```python
from build123d import *

# Parameters (mm, degrees)
SKETCH2_W           = 124.173
SKETCH2_H           = 119.38
BOSS_EXTRUDE1_DEPTH = 3.175
SKETCH4_R           = 1.905
CUT_EXTRUDE1_DEPTH  = 14.175
SKETCH10_W          = 1.59
SKETCH10_H          = 120
CUT_EXTRUDE3_DEPTH  = 10
SKETCH11_R          = 1.905
CUT_EXTRUDE4_DEPTH  = 10


with BuildPart() as part:
    # Sketch2 → Boss-Extrude1 (new body)
    with BuildSketch(Plane.XY):
        with Locations((40.767155738, -50.87039032)):
            Rectangle(SKETCH2_W, SKETCH2_H)
    extrude(amount=BOSS_EXTRUDE1_DEPTH)

    # Sketch4 → Cut-Extrude1 (cut)
    with BuildSketch(Plane.XY):
        with Locations((-15.867344262, -37.32039032)):
            Circle(SKETCH4_R)
        with Locations((-15.867344262, -64.42239032)):
            Circle(SKETCH4_R)
        with Locations((84.503655738, 3.36760968)):
            Circle(SKETCH4_R)
        with Locations((84.503655738, -105.10839032)):
            Circle(SKETCH4_R)
    extrude(amount=CUT_EXTRUDE1_DEPTH, mode=Mode.SUBTRACT)

    # Sketch10 → Cut-Extrude3 (cut)
    with BuildSketch(Plane(origin=(102.853655738, 0, 0), x_dir=(0, 0, -1), z_dir=(1, 0, 0))):
        with Locations((-2.380000064, -51.180389625)):
            Rectangle(SKETCH10_W, SKETCH10_H)
    extrude(amount=-CUT_EXTRUDE3_DEPTH, mode=Mode.SUBTRACT)

    # Sketch11 → Cut-Extrude4 (cut)
    with BuildSketch(Plane.XY.offset(1.585000064)):
        with Locations((97.853655738, -9.260389625)):
            Circle(SKETCH11_R)
        with Locations((97.853655738, -27.350389625)):
            Circle(SKETCH11_R)
        with Locations((97.853655738, -45.430389625)):
            Circle(SKETCH11_R)
        with Locations((97.853655738, -96.56039032)):
            Circle(SKETCH11_R)
    extrude(amount=-CUT_EXTRUDE4_DEPTH, mode=Mode.SUBTRACT)


solid = part.part
```
Geometry check sheet. Reference: the model listing, model coordinates, mm. A direction names the side the tool comes from. Give positions to 0.01 mm unless a question says otherwise; leave off trailing zeros. Write each loop counter-clockwise with the first axis right and the second up, starting at its lowest first coordinate (ties: lowest second). Pieces come first, ordered by that corner, then holes. Notation, with made-up numbers: (76, 38) - (124, 38) arc R28 ccw to (124, 64) - close; hole circle Ø8 at (63, -25). An arc over 180 degrees is marked (long way). Use a Markdown table: item, result.
Q1. Section check B-B, the plane y = -33. Enter the section's corners in (x, z) (3 decimals), then the cut area to 3 significant figures.
Computed:
| item | result |
|---|---|
| outline | (-21.319, 0) - (102.854, 0) - (102.854, 1.585) - (92.854, 1.585) - (92.854, 3.175) - (-21.319, 3.175) - close |
| area | 378 mm² |
Q2. Thickness scan on L1, parallel to X at y = -37, z = 2; L2, parallel to X at y = -9, z = 0.35; L3, parallel to Y at x = -15.5, z = 0.85. Record the ranges inside material, lowest first. Write a range as [from, to].
Computed:
| item | result |
|---|---|
| L1 | x = [-21.32, -17.75], [-13.99, 92.85] |
| L2 | x = [-21.32, 95.97], [99.74, 102.85] |
| L3 | y = [-110.56, -66.29], [-62.55, -39.19], [-35.45, 8.82] |
Q3. Set-up check for faces 1 (the face through (40, 8.82, 2)), 2 (the face through (98, -52, 1.585)): record each of +Z, -Z, +X, -X, +Y, -Y from which the full face is reachable in a straight line by a thin tool's end or side.
Computed:
| item | result |
|---|---|
| face 1 | +Z, -Z, +X, -X, +Y |
| face 2 | +Z, +X, +Y, -Y |
Q4. Go/stop test with flat-tipped pins: P1, Ø1.7, axis at y = -26.5, z = 2.5, coming from the +X side; P2, Ø6, axis at x = 97.85, y = -27.35, coming from the +Z side (3 decimals). Record where each tip stops, or that it passes through.
Computed:
| item | result |
|---|---|
| P1 | stops at x = 92.85 |
| P2 | stops at z = 1.585 |
Q5. Section check A-A, the plane z = 2.15. Enter the section's corners in (x, y) (3 decimals).
Computed:
| item | result |
|---|---|
| outline | (-21.319, -110.56) - (92.854, -110.56) - (92.854, 8.82) - (-21.319, 8.82) - close; hole circle Ø3.81 at (-15.867, -64.422); hole circle Ø3.81 at (-15.867, -37.32); hole circle Ø3.81 at (84.504, -105.108); hole circle Ø3.81 at (84.504, 3.368) |
